from build123d import *

# Parameters (mm, degrees)
F0_R     = 4.1
F1_DEPTH = 10
F2_R     = 30
F3_ANGLE = 90


with BuildPart() as f1:
    # F0 (on Top) → F1 (new body)
    with BuildSketch(Plane.XY):
        Polygon((-265, 45), (-300, 45), (-300, -45), (-265, -45), (-265, -40), (-255, -40), (-255, -45), (255, -45), (255, -40), (265, -40), (265, -45), (300, -45), (300, 45), (265, 45), (265, 40), (255, 40), (255, 50), (-255, 50), (-255, 40), (-265, 40), align=None)
        with Locations((-282.5, 0)):
            Circle(F0_R, mode=Mode.SUBTRACT)
        with Locations((282.5, 0)):
            Circle(F0_R, mode=Mode.SUBTRACT)
    extrude(amount=F1_DEPTH)

    # F2
    f2_edges = [f1.edges().sort_by_distance(p)[0] for p in [
        (-300, -45, 5),
        (-300, 45, 5),
        (300, 45, 5),
        (300, -45, 5),
    ]]
    fillet(f2_edges, radius=F2_R)


with BuildPart() as f1_1:
    # F3: moved
    add(f1.part.rotate(Axis((282.5, -45, 0), (1, 0, 0)), F3_ANGLE))


solid = f1_1.part
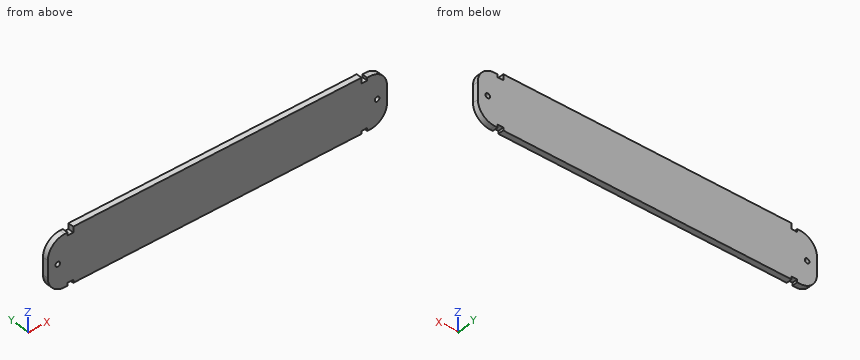
The listing builds one solid part. Answer for the finished solid, in the listing's coordinates (mm). Coordinates: 2 decimals unless noted, no trailing zeros. Write each loop counter-clockwise with the first axis right and the second up, starting at its lowest first coordinate (ties: lowest second). Pieces come first, ordered by that corner, then holes. Notation, with made-up numbers: M 4.5,89.5 L 9.5,89.5 A24 cw 9.5,118.5 Z; hole C 13,18.5 d1. An arc over 180 degrees is marked long. Use one line per item in the form item = value.
Item 1: Find section A-A, the plane y = -50.75. Give the vertices of the cut face in (x, z).
Model answer:
outline = M -300,30 A30 ccw -270,0 L -265,0 L -265,5 L -255,5 L -255,0 L 255,0 L 255,5 L 265,5 L 265,0 L 270,0 A30 ccw 300,30 L 300,60 A30 ccw 270,90 L 265,90 L 265,85 L 255,85 L 255,95 L -255,95 L -255,85 L -265,85 L -265,90 L -270,90 A30 ccw -300,60 Z; hole C -282.5,45 d8.2; hole C 282.5,45 d8.2
Item 2: Find the intervals of material crossed by probe 1 along Z at (x, y) = (282.5, -50.75); probe 2 along X at (y, z) = (-51, 76); probe 3 along X at (y, z) = (-50, 27.5), in increasing order.
Model answer:
probe_1 = 2.73 to 40.9, 49.1 to 87.27
probe_2 = -295.38 to 295.38
probe_3 = -299.9 to 299.9
Item 3: Given P1, Ø4, axis at y = -50.5, z = 1.5, coming from the +X side; P2, Ø2.5, axis at y = -51, z = 87, coming from the +X side; P3, Ø2.5, axis at x = -268.5, y = -51, coming from the +Z side; P4, Ø10.5, axis at x = -282.5, z = 45, coming from the -Y side, each flat-ended and moving along its own axis, determine where each tip first touches the part or whether it passes through.
Model answer:
P1 = 284.06
P2 = 285.39
P3 = 90
P4 = -55
